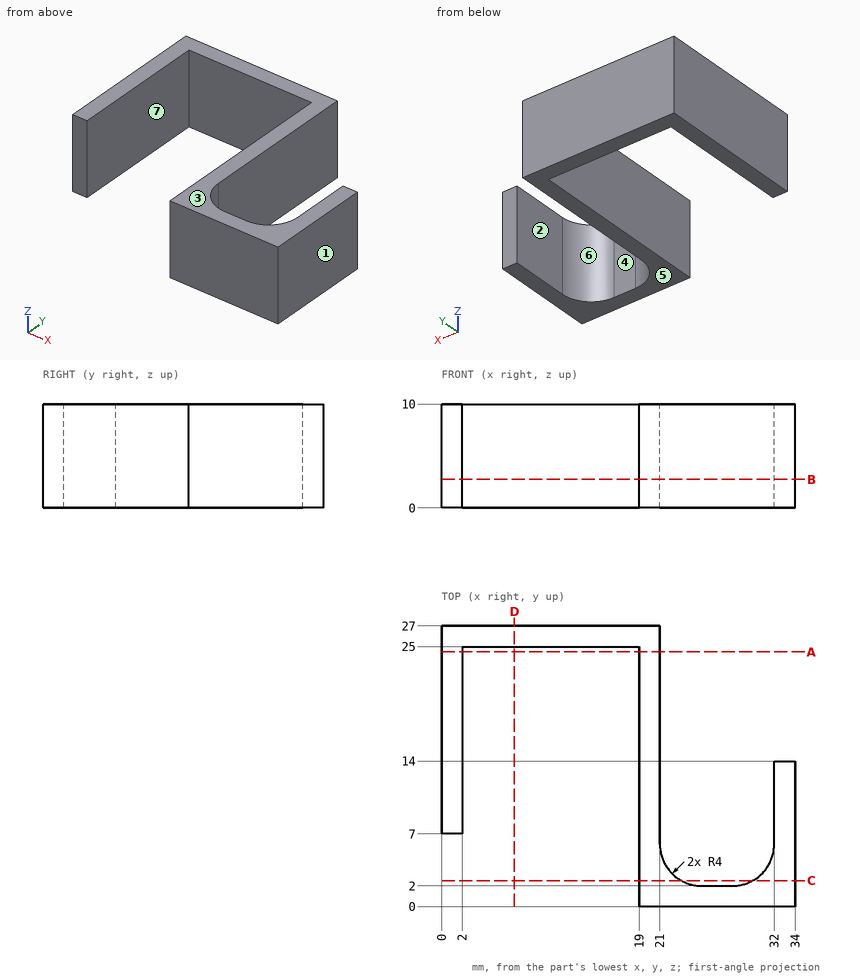
Part print with two shaded views. Sizes in mm from the minimum x, y, z corner. A direction names the side the tool comes from. Round coordinates to 2 decimals unless told otherwise and drop trailing zeros. Order: outer loops, then holes, each group sorted by start corner. A loop starts at its lowest first (then second) coordinate and runs counter-clockwise, first axis right, second up. Notation, with made-up numbers: (-12, 29.5) - (1, 29.5) arc R20 ccw to (1, 63.5) - close; hole circle Ø9 at (-35.75, -28). An arc over 180 degrees is marked (long way). Return JSON: item names as keys, results as strings.
(1) Wall check: probe 1 along X at (y, z) = (11.75, 7); probe 2 along X at (y, z) = (6.25, 9); probe 3 along X at (y, z) = (15, 8.25). Give the ranges that are in metal, low to high. Write a range as from..to.
Answer key:
{"probe 1": "x = 0..2, 19..21, 32..34", "probe 2": "x = 19..21, 32..34", "probe 3": "x = 0..2, 19..21"}
(2) Cut at C-C (y = 2.5). Give the cut face in (x, z), then the cut area to 3 significant figures.
Answer key:
{"outline": "(19, 0) - (23.06, 0) - (23.06, 10) - (19, 10) - close; (29.94, 0) - (34, 0) - (34, 10) - (29.94, 10) - close", "area": "81.3 mm^2"}
(3) Pin check, flat tips, straight feed: pin 1 Ø2.5 at (x, z) = (26.5, 7.5) entering from +Y; pin 2 Ø10 at (x, y) = (19, 12.5) entering from -Z; pin 3 Ø0.6 at (x, z) = (33.5, 6) entering from +Y; pin 4 Ø5 at (x, z) = (12, 6.5) entering from -Y. Stop position of each tip, or through.
Answer key:
{"pin 1": "stops at y = 2", "pin 2": "stops at z = 0", "pin 3": "stops at y = 14", "pin 4": "stops at y = 25"}
(4) Cut at B-B (z = 2.75). Give the cut face in (x, y).
Answer key:
{"outline": "(0, 7) - (2, 7) - (2, 25) - (19, 25) - (19, 0) - (34, 0) - (34, 14) - (32, 14) - (32, 6) arc R4 cw to (28, 2) - (25, 2) arc R4 cw to (21, 6) - (21, 27) - (0, 27) - close"}
(5) Cut at D-D (x = 7). Give the cut face in (y, z).
Answer key:
{"outline": "(25, 0) - (27, 0) - (27, 10) - (25, 10) - close"}
(6) Pull direction X, two halves, no side cores. Call the marked faces 1, 2, 3 and 4: +X half, -X half, draft (parallel to the pull), parting line (faces both ways), or undercut.
Answer key:
{"face 1": "+X half", "face 2": "undercut", "face 3": "draft", "face 4": "undercut"}
(7) Tool access for the marked faces 5, 6 and 7: list every direction of +Z, -Z, +X, -X, +Y, -Y with a clear straight run to the whole face (end or side of a thin tool).
Answer key:
{"face 5": "-Z, +X, -X, +Y, -Y", "face 6": "+Z, -Z, +Y", "face 7": "+Z, -Z, -Y"}
(8) Cut at A-A (y = 24.5). Give the cut face in (x, z), then the cut area to 3 significant figures.
Answer key:
{"outline": "(0, 0) - (2, 0) - (2, 10) - (0, 10) - close; (19, 0) - (21, 0) - (21, 10) - (19, 10) - close", "area": "40.0 mm^2"}
